Geometry: final body of the model. Coordinates: model frame, mm. A direction names the side the tool comes from. Give positions to 0.01 mm unless a question says otherwise; leave off trailing zeros. Loops run counter-clockwise (first coordinate to the right, second up) from the corner with the lowest first, then second, coordinate; pieces in that order, holes last. Notation, with made-up numbers: (65, -13.5) -> (72, -13.5) arc R16 cw to (72, 2.5) -> close; hole circle Ø2 at (-2, 85.5). An arc over 180 degrees is marked (long way). Answer in a Markdown table with one row per item. Add a question column.
from build123d import *

# Parameters (mm, degrees)
SKETCH1_R           = 2.1
BOSS_EXTRUDE2_DEPTH = 1.8


with BuildPart() as part:
    # Sketch1 → Boss-Extrude2 (new body)
    with BuildSketch(Plane.YZ):
        with BuildLine():
            Line((-2.6, 0), (-2.6, -5.1875))
            Line((-2.6, -5.1875), (-1.1, -5.1875))
            Line((-1.1, -5.1875), (-1.1, -2.355843798))
            ThreePointArc((-1.1, -2.355843798), (0.024387933, -2.599885618), (1.144, -2.334794209))
            Line((1.144, -2.334794209), (1.1, -5.1875))
            Line((1.1, -5.1875), (2.6, -5.1875))
            Line((2.6, -5.1875), (2.6, 0))
            ThreePointArc((2.6, 0), (0, 2.6), (-2.6, 0))
        make_face()
        with Locations(Location((0, 0, 0), (0, 0, 270))):
            Circle(SKETCH1_R, mode=Mode.SUBTRACT)
    extrude(amount=BOSS_EXTRUDE2_DEPTH)


solid = part.part
(1) Cut plane B-B on z = -4.5. Return the cut outline in (x, y), then the cut area to 3 significant figures.
(2) Material intervals for line 1 along Z through (x, y) = (0.35, -0.05); line 2 along Z through (x, y) = (1.55, -0.8); line 3 along Y through (x, z) = (0.5, 1.25), sorted ascending. Write a range as from..to.
(3) Draft query along Z for faces 3 (the flat face through (1, 2, -5.188)), 4 (the flat face through (1.8, -1.2, -2.1)), 5 (the cylindrical face through (0.887, 0.631, -2.003)). Return one class per face: +Z half, -Z half, draft (parallel to the pull), parting line (faces both ways), or undercut.
(4) Cut plane A-A on y = 0. Return the cut outline in (x, z), then the cut area to 3 significant figures.
(5) Cut plane C-C on x = 1.45. Return the cut outline in (y, z).
(6) Reachability of faces 1 (the flat face through (1, -2.6, -3)), 2 (the flat face through (1, -1.1, -4)) from +Z, -Z, +X, -X, +Y, -Y: full face, straight path, thin tool, end or side. Return the list, or none.
(7) Cut plane D-D on y = -2.25. Return the cut outline in (x, z).
Answer list:
| question | item | result |
|---|---|---|
| 1 | outline | (0, -2.6) -> (1.8, -2.6) -> (1.8, -1.1) -> (0, -1.1) -> close; (0, 1.11) -> (1.8, 1.11) -> (1.8, 2.6) -> (0, 2.6) -> close |
| 1 | area | 5.38 mm² |
| 2 | line 1 | z = -2.6..-2.1, 2.1..2.6 |
| 2 | line 2 | z = -2.47..-1.94, 1.94..2.47 |
| 2 | line 3 | y = -2.28..-1.69, 1.69..2.28 |
| 3 | face 3 | -Z half |
| 3 | face 4 | draft |
| 3 | face 5 | undercut |
| 4 | outline | (0, -2.6) -> (1.8, -2.6) -> (1.8, -2.1) -> (0, -2.1) -> close; (0, 2.1) -> (1.8, 2.1) -> (1.8, 2.6) -> (0, 2.6) -> close |
| 4 | area | 1.80 mm² |
| 5 | outline | (-2.6, -5.19) -> (-1.1, -5.19) -> (-1.1, -2.36) arc R2.6 ccw to (1.14, -2.33) -> (1.1, -5.19) -> (2.6, -5.19) -> (2.6, 0) arc R2.6 ccw to (-2.6, 0) -> close; hole circle Ø4.2 at (0, 0) |
| 6 | face 1 | +Z, -Z, +X, -X, -Y |
| 6 | face 2 | -Z, +X, -X |
| 7 | outline | (0, -5.19) -> (1.8, -5.19) -> (1.8, 1.3) -> (0, 1.3) -> close |
